```python
from build123d import *

# Parameters (mm, degrees)
ESQUISSE1_W        = 156
ESQUISSE1_H        = 42.000000092
BOSS_EXTRU_1_DEPTH = 3


with BuildPart() as part:
    # Esquisse1 → Boss.-Extru.1 (new body)
    with BuildSketch(Plane.XY):
        with BuildLine():
            Line((0, 0), (0, 10))
            Line((0, 10), (3, 10))
            Line((3, 10), (3, 30))
            Line((3, 30), (0, 30))
            Line((0, 30), (0, 50))
            Line((0, 50), (3, 50))
            Line((3, 50), (3, 70))
            Line((3, 70), (0, 70))
            Line((0, 70), (0, 80))
            Line((0, 80), (-13, 80))
            Line((-13, 80), (-13, 83))
            Line((-13, 83), (-33, 83))
            Line((-33, 83), (-33, 80))
            Line((-33, 80), (-73, 80))
            Line((-73, 80), (-73, 83))
            Line((-73, 83), (-93, 83))
            Line((-93, 83), (-93, 80))
            Line((-93, 80), (-133, 80))
            Line((-133, 80), (-133, 83))
            Line((-133, 83), (-153, 83))
            Line((-153, 83), (-153, 80))
            Line((-153, 80), (-166, 80))
            Line((-166, 80), (-166, 70))
            Line((-166, 70), (-169, 70))
            Line((-169, 70), (-169, 50))
            Line((-169, 50), (-166, 50))
            Line((-166, 50), (-166, 30))
            Line((-166, 30), (-169, 30))
            Line((-169, 30), (-169, 10))
            Line((-169, 10), (-166, 10))
            Line((-166, 10), (-166, 0))
            Line((-166, 0), (-153, 0))
            Line((-153, 0), (-153, -3))
            Line((-153, -3), (-133, -3))
            Line((-133, -3), (-133, 0))
            Line((-133, 0), (-92.99999998, 0))
            add(Edge.make_bspline(
                [(-92.99999998, 0), (-83, 59.999999815), (-73.00000002, 0)],
                knots=[0, 0, 0, 1, 1, 1], degree=2))
            Line((-73.00000002, 0), (-33, 0))
            Line((-33, 0), (-33, -3))
            Line((-33, -3), (-13, -3))
            Line((-13, -3), (-13, 0))
            Line((-13, 0), (0, 0))
        make_face()
        with Locations((-83, 53.999999954)):
            Rectangle(ESQUISSE1_W, ESQUISSE1_H, mode=Mode.SUBTRACT)
    extrude(amount=BOSS_EXTRU_1_DEPTH)


solid = part.part
```
The listing builds one solid part. Answer for the finished solid, in the listing's coordinates (mm). A direction names the side the tool comes from. Coordinates: 2 decimals unless noted, no trailing zeros. Loops run counter-clockwise (first coordinate to the right, second up) from the corner with the lowest first, then second, coordinate; pieces in that order, holes last. Notation, with made-up numbers: M -4,46 L 55,46 A3 ccw 55,51 Z; hole C 30.25,77.25 d6. An arc over 180 degrees is marked long. Answer as a JSON object with one key per item and string values. Group by question number.
Item 1: Each of these flat-tipped pins is pushed along its axis until it touches: P1, Ø0.9, axis at x = 1.5, z = 2, coming from the +Y side; P2, Ø0.9, axis at x = -167.5, z = 2, coming from the -Y side; P3, Ø0.9, axis at x = -157, z = 1, coming from the +Y side. Where does it stop, or does it pass through?
Item 2: Determine the mould class of faces 5 (the face through (-169, 60, 1)), 6 (the face through (-53, 0, 1)), 7 (the face through (1, 50, 1)) for opening direction Y: +Y half, -Y half, draft (parallel to the pull), parting line (faces both ways), or undercut.
Item 3: Consider L1, parallel to X at y = 80.5, z = 2.65; L2, parallel to Y at x = -111, z = 0.35; L3, parallel to X at y = 70.5, z = 0.75. Determine where each line is inside the solid, lowest interval first.
Item 4: Section A-A (y = 47) is taken. Write down the section's boundary in (x, z), and give its area (3 significant figures).
Item 5: Which of the six approach directions +Z, -Z, +X, -X, +Y, -Y give full straight-line access (tool end or side, diameter ignored) to faces 1 (the face through (2, 30, 1)), 2 (the face through (-33, -1, 1)), 3 (the face through (-53, 80, 1)), 4 (the face through (0, 75, 1))?
Item 6: Section B-B (x = -70) is taken. Write down the section's boundary in (y, z), and give its area (3 significant figures).
Solved:
{
 "1": {"P1": "stops at y = 70", "P2": "stops at y = 10", "P3": "stops at y = 80"},
 "2": {"face 5": "draft", "face 6": "-Y half", "face 7": "undercut"},
 "3": {"L1": "x = -153 to -133, -93 to -73, -33 to -13", "L2": "y = 0 to 33, 75 to 80", "L3": "x = -166 to -161, -5 to 0"},
 "4": {"outline": "M -166,0 L -161,0 L -161,3 L -166,3 Z; M -5,0 L 0,0 L 0,3 L -5,3 Z", "area": "30.0 mm2"},
 "5": {"face 1": "+Z, -Z, +X", "face 2": "+Z, -Z, -Y", "face 3": "+Z, -Z, +Y", "face 4": "+Z, -Z, +X, +Y"},
 "6": {"outline": "M 0,0 L 33,0 L 33,3 L 0,3 Z; M 75,0 L 80,0 L 80,3 L 75,3 Z", "area": "114 mm2"}
}
